```python
from build123d import *

# Parameters (mm, degrees)
CROQUIS1_R                = 1.5
SALIENTE_EXTRUIR1_DEPTH   = 4
CROQUIS2_R                = 2.9
CORTAR_EXTRUIR1_DEPTH     = 2
SALIENTE_EXTRUIR2_DEPTH   = 65
CORTAR_EXTRUIR2_OUTLINE_W = 7.281077338
CORTAR_EXTRUIR2_OUTLINE_H = 8.780929931
CORTAR_EXTRUIR2_DEPTH     = 8.6
CORTAR_EXTRUIR2_TAPER     = -65
CROQUIS5_W                = 41.142355125
CROQUIS5_H                = 35.377069929
CORTAR_EXTRUIR3_DEPTH     = 10
SALIENTE_EXTRUIR3_DEPTH   = 7
CORTAR_EXTRUIR4_DEPTH     = 5
CORTAR_EXTRUIR5_START     = -7
CROQUIS8_W                = 2.5
CROQUIS8_H                = 1.5
CORTAR_EXTRUIR5_DEPTH     = 7
CORTAR_EXTRUIR6_DEPTH     = 10
SALIENTE_EXTRUIR4_DEPTH   = 3.7
SALIENTE_EXTRUIR5_DEPTH   = 2.558793
CORTAR_EXTRUIR7_DEPTH     = 10
SALIENTE_EXTRUIR6_DEPTH   = 2
CROQUIS15_W               = 4
CROQUIS15_H               = 4
SALIENTE_EXTRUIR7_DEPTH   = 1
CROQUIS16_R               = 1.4
CORTAR_EXTRUIR8_DEPTH     = 1


# Read off the part's stored shape, not the designer's step: Cortar-Extruir2
with BuildPart() as part:
    # Croquis1 → Saliente-Extruir1 (new body)
    with BuildSketch(Plane.XY):
        with BuildLine():
            Line((-55.370631899, 7.045687646), (-55.370631899, 3.345687646))
            ThreePointArc((-55.370631899, 3.345687646), (-61.070631899, -0.995420457), (-66.770631899, 3.345687646))
            Line((-66.770631899, 3.345687646), (-66.770631899, 7.045687646))
            ThreePointArc((-66.770631899, 7.045687646), (-61.070631899, 12.745687646), (-55.370631899, 7.045687646))
        make_face()
        with Locations((-61.070631899, 7.045687646)):
            Circle(CROQUIS1_R, mode=Mode.SUBTRACT)
    extrude(amount=SALIENTE_EXTRUIR1_DEPTH)

    # Croquis2 → Cortar-Extruir1 (cut)
    with BuildSketch(Plane.XY.offset(4)):
        with Locations((-61.070631899, 7.045687646)):
            Circle(CROQUIS2_R)
    extrude(amount=-CORTAR_EXTRUIR1_DEPTH, mode=Mode.SUBTRACT)

    # Croquis3 → Saliente-Extruir2 (add)
    with BuildSketch(Plane.XY.offset(4)):
        with BuildLine():
            Line((-63.970631899, 7.045687646), (-66.770631899, 7.045687646))
            Line((-66.770631899, 7.045687646), (-66.770631899, 3.345687646))
            ThreePointArc((-66.770631899, 3.345687646), (-61.070631899, -0.995420457), (-55.370631899, 3.345687646))
            Line((-55.370631899, 3.345687646), (-55.370631899, 7.045687646))
            Line((-55.370631899, 7.045687646), (-58.170631899, 7.045687646))
            ThreePointArc((-58.170631899, 7.045687646), (-61.070631899, 4.145687646), (-63.970631899, 7.045687646))
        make_face()
    extrude(amount=SALIENTE_EXTRUIR2_DEPTH)

    # Cortar-Extruir2 outline → Cortar-Extruir2 (cut)
    with BuildSketch(Plane.YZ.offset(-58.170631899)):
        with Locations((3.405148977, 64.609535034)):
            Rectangle(CORTAR_EXTRUIR2_OUTLINE_W, CORTAR_EXTRUIR2_OUTLINE_H)
    extrude(amount=-CORTAR_EXTRUIR2_DEPTH, taper=CORTAR_EXTRUIR2_TAPER, mode=Mode.SUBTRACT)

    # Croquis5 → Cortar-Extruir3 (cut)
    with BuildSketch(Plane(origin=(-70.846238664, 0, 33.03614364), x_dir=(0.422618261740701, 0, 0.9063077870366493), z_dir=(-0.9063077870366493, 1.4037441023509523e-15, 0.422618261740701))):
        with Locations((23.845262034, -3.548141358)):
            Rectangle(CROQUIS5_W, CROQUIS5_H)
    extrude(amount=CORTAR_EXTRUIR3_DEPTH, mode=Mode.SUBTRACT)

    # Croquis6 → Saliente-Extruir3 (add)
    with BuildSketch(Plane(origin=(-70.846238664, 0, 33.03614364), x_dir=(0.422618261740701, 0, 0.9063077870366493), z_dir=(-0.9063077870366493, 1.4037441023509523e-15, 0.422618261740701))):
        with BuildLine():
            Line((31.131056203, 7.045687646), (29.993040795, 7.045687646))
            add(Edge.make_bspline(
                [(16.269071612, 7.045687646), (16.269071612, 4.145687646), (23.131056203, 4.145687646), (29.993040795, 4.145687646), (29.993040795, 7.045687646)],
                knots=[3.141592654, 3.141592654, 3.141592654, 4.71238898, 4.71238898, 6.283185307, 6.283185307, 6.283185307], degree=2, weights=[1, 0.707106781, 1, 0.707106781, 1]))
            Line((16.269071612, 7.045687646), (15.131056203, 7.045687646))
            Line((15.131056203, 7.045687646), (15.131056203, -13.654312354))
            Line((15.131056203, -13.654312354), (31.131056203, -13.654312354))
            Line((31.131056203, -13.654312354), (31.131056203, 7.045687646))
        make_face()
    extrude(amount=SALIENTE_EXTRUIR3_DEPTH)

    # Croquis7 → Cortar-Extruir4 (cut)
    with BuildSketch(Plane(origin=(-77.190393173, 0, 35.994471473), x_dir=(0.42261826174070094, 0, 0.9063077870366492), z_dir=(-0.9063077870366493, 1.403744102350952e-15, 0.422618261740701))):
        with BuildLine():
            Line((25.381056203, 4.145687646), (26.731056203, -3.854312354))
            Line((26.731056203, -3.854312354), (31.131056203, -3.854312354))
            Line((31.131056203, -3.854312354), (31.131056203, -10.654312354))
            Line((31.131056203, -10.654312354), (15.131056203, -10.654312354))
            Line((15.131056203, -10.654312354), (15.131056203, -3.854312354))
            Line((15.131056203, -3.854312354), (19.531056203, -3.854312354))
            Line((19.531056203, -3.854312354), (20.881056203, 4.145687646))
            Line((20.881056203, 4.145687646), (20.881056203, 4.306015013))
            add(Edge.make_bspline(
                [(20.881056203, 4.306015013), (23.131056203, 3.97597782), (25.381056203, 4.306015013)],
                knots=[4.378316067, 4.378316067, 4.378316067, 5.046461894, 5.046461894, 5.046461894], degree=2, weights=[1, 0.944714701, 1]))
            Line((25.381056203, 4.306015013), (25.381056203, 4.145687646))
        make_face()
    extrude(amount=-CORTAR_EXTRUIR4_DEPTH, mode=Mode.SUBTRACT)

    # Croquis8 → Cortar-Extruir5 (cut)
    with BuildSketch(Plane(origin=(-77.190393173, 0, 35.994471473), x_dir=(0.42261826174070094, 0, 0.9063077870366492), z_dir=(-0.9063077870366493, 1.403744102350952e-15, 0.422618261740701)).offset(CORTAR_EXTRUIR5_START)):
        with Locations((17.381056203, -2.104312354)):
            Rectangle(CROQUIS8_W, CROQUIS8_H)
        with Locations((28.881056203, -2.104312354)):
            Rectangle(CROQUIS8_W, CROQUIS8_H)
    extrude(amount=CORTAR_EXTRUIR5_DEPTH, mode=Mode.SUBTRACT)

    # Croquis9 → Cortar-Extruir6 (cut)
    with BuildSketch(Plane(origin=(0, 7.045687646, 0), x_dir=(1, 0, 0), z_dir=(0, 1, 0))):
        Polygon((-57.689685805, -61.250462296), (-55.370631899, -60.1690697), (-55.370631899, -66.223689447), align=None)
    extrude(amount=-CORTAR_EXTRUIR6_DEPTH, mode=Mode.SUBTRACT)

    # Croquis10 → Saliente-Extruir4 (add)
    with BuildSketch(Plane(origin=(0, 7.045687646, 0), x_dir=(1, 0, 0), z_dir=(0, 1, 0))):
        Polygon((-66.770631899, -41.776310553), (-66.770631899, -47.8309303), (-64.451577993, -46.749537704), align=None)
    extrude(amount=-SALIENTE_EXTRUIR4_DEPTH)

    # Croquis12 → Saliente-Extruir5 (add)
    with BuildSketch(Plane(origin=(-70.846238664, 0, 33.03614364), x_dir=(0.422618261740701, 0, 0.9063077870366493), z_dir=(-0.9063077870366493, 1.4037441023509523e-15, 0.422618261740701))):
        with BuildLine():
            Line((15.131056203, 3.345687646), (15.131056203, 0.066589345))
            ThreePointArc((15.131056203, 0.066589345), (12.129139109, 1.273987016), (9.64370718, 3.345687646))
            Line((9.64370718, 3.345687646), (15.131056203, 3.345687646))
        make_face()
    extrude(amount=SALIENTE_EXTRUIR5_DEPTH)

    # Croquis13 → Cortar-Extruir7 (cut)
    with BuildSketch(Plane(origin=(0, 3.345687646, 0), x_dir=(1, 0, 0), z_dir=(0, 1, 0))):
        Polygon((-66.770631899, -47.8309303), (-66.770631899, -41.776310553), (-69.089685805, -42.857703149), align=None)
    extrude(amount=-CORTAR_EXTRUIR7_DEPTH, mode=Mode.SUBTRACT)

    # Croquis14 → Saliente-Extruir6 (add)
    with BuildSketch(Plane(origin=(0, 0, 0), x_dir=(-1, 0, 0), z_dir=(0, 0, -1))):
        Polygon((66.770631899, 3.345687646), (70.770631899, 3.345687646), (70.770631899, 0.345687646), (66.770631899, 0.345687646), (66.770631899, -0.854312354), (71.970631899, -0.854312354), (71.970631899, 4.545687646), (66.770631899, 4.545687646), align=None)
    extrude(amount=-SALIENTE_EXTRUIR6_DEPTH)

    # Croquis15 → Saliente-Extruir7 (add)
    with BuildSketch(Plane.XZ.offset(-3.345687646)):
        with Locations((-68.770631899, 0)):
            Rectangle(CROQUIS15_W, CROQUIS15_H)
    extrude(amount=SALIENTE_EXTRUIR7_DEPTH)

    # Croquis16 → Cortar-Extruir8 (cut)
    with BuildSketch(Plane.XZ.offset(-2.345687646)):
        with Locations((-68.770631899, -2)):
            Circle(CROQUIS16_R)
    extrude(amount=-CORTAR_EXTRUIR8_DEPTH, mode=Mode.SUBTRACT)


solid = part.part
```
The model under review builds one solid part; all positions refer to its coordinate system, in mm. A direction names the side the tool comes from. Round coordinates to 2 decimals unless told otherwise and drop trailing zeros. Write each loop counter-clockwise with the first axis right and the second up, starting at its lowest first coordinate (ties: lowest second). Pieces come first, ordered by that corner, then holes. Notation, with made-up numbers: (-11.5, -13.5) - (21.5, -13.5) arc R35 cw to (21.5, 19.5) - close; hole circle Ø2 at (53, 11). An arc over 180 degrees is marked (long way). One line per question, with ' | ' between items.
Item 1: For P1, Ø12, axis at y = 8, z = 51.5, coming from the -X side; P2, Ø2, axis at x = -69.5, z = -1.5, coming from the +Y side; P3, Ø0.6, axis at y = 0, z = 1.5, coming from the +X side; P4, Ø1, axis at y = 8.5, z = 34.5, coming from the -X side, all flat-tipped, find the tip position at first contact; note any pin that passes through.
Resolved:
P1: stops at x = -70.8 | P2: stops at y = 3.35 | P3: stops at x = -57.38 | P4: passes through
Item 2: Add section A-A, the plane z = 33.5. Give the boundary of the cut face in (x, y).
Resolved:
outline: (-66.77, 3.35) arc R5.91 ccw to (-55.37, 3.35) - (-55.37, 7.05) - (-58.17, 7.05) arc R2.9 cw to (-63.97, 7.05) - (-66.77, 7.05) - close
Item 3: Add section B-B, the plane y = -11.5. Give the boundary of the cut face in (x, z), then the cut area to 3 significant figures.
Resolved:
outline: (-70.8, 49.71) - (-64.45, 46.75) - (-57.69, 61.25) - (-64.03, 64.21) - close | area: 112 mm2
Item 4: To check wall thickness, follow probe 1 along Y at (x, z) = (-61, 13.5) (3 decimals); probe 2 along Z at (x, y) = (-58.25, 11.25); probe 3 along X at (y, z) = (5.5, 38). State the ranges of each line that lie inside material, in increasing order.
Resolved:
probe 1: y = -0.995 to 4.147 | probe 2: z = 0 to 4 | probe 3: x = -66.77 to -63.52, -58.62 to -55.37
Item 5: The part is to be moulded in two halves that separate along Z. For faces 4 (the face through (-67.46, -12.13, 56.86)), 5 (the face through (-71.971, 2, 1)), 6 (the face through (-67, -1.354, 50)), 7 (the face through (-67, -2.854, 50)), say which applies: pulls with the +Z half, pulls with the -Z half, needs draft (parallel to the pull), parting line crosses it, or undercut.
Resolved:
face 4: pulls with the +Z half | face 5: needs draft | face 6: undercut | face 7: undercut
Item 6: For faces 1 (the face through (-66, 7.046, 27)), 2 (the face through (-69, 0.346, 1)), 3 (the face through (-69, -0.854, 1)), list the 3-axis set-ups (+Z, -Z, +X, -X, +Y, -Y) from which the entire face can be reached by the end or side of a thin tool; tool diameter is ignored.
Resolved:
face 1: +Z, +X, -X, +Y | face 2: -Z | face 3: -Z, -X, -Y
